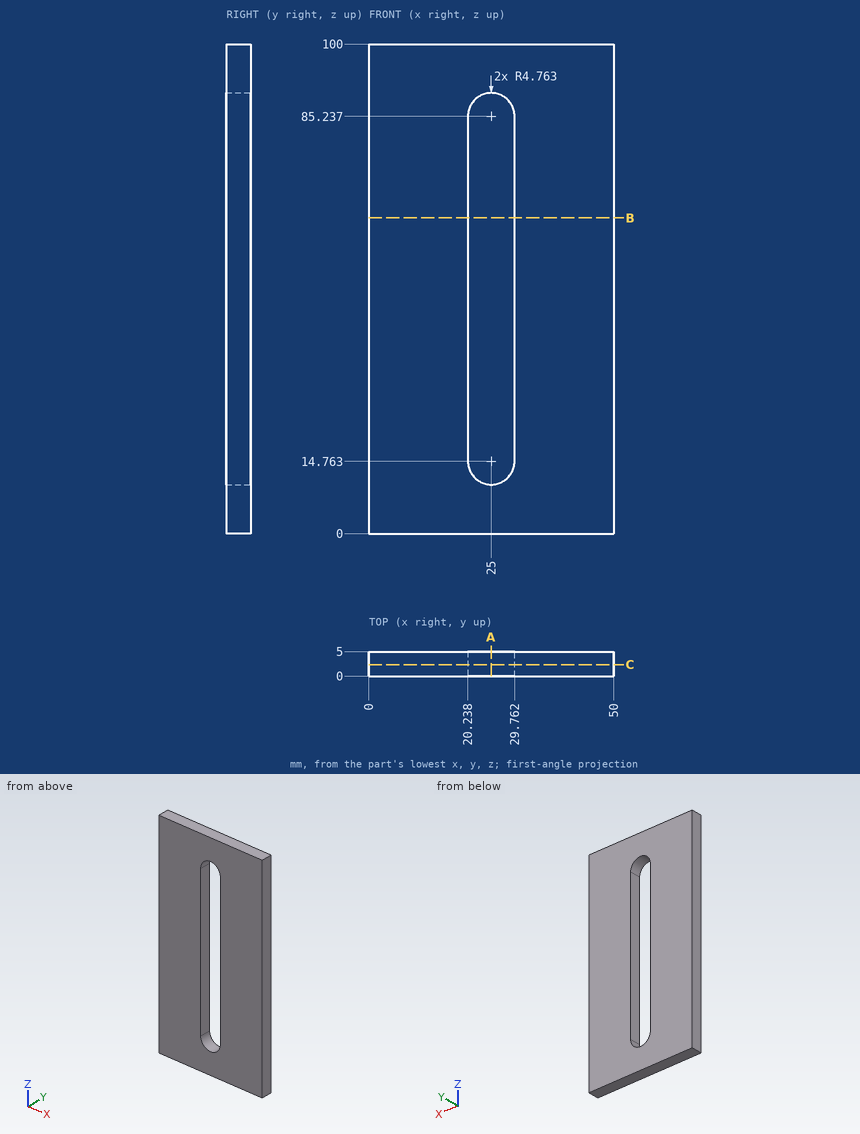
Geometry check sheet. Reference: drawing and pictorial views, mm from the part's lowest x, y, z. Round coordinates to 2 decimals unless told otherwise and drop trailing zeros. Order: outer loops, then holes, each group sorted by start corner. A loop starts at its lowest first (then second) coordinate and runs counter-clockwise, first axis right, second up. Notation, with made-up numbers: M -26,57 L 2,57 A15 cw 2,61 Z; hole C -22.5,9.5 d7. An arc over 180 degrees is marked long. Write item = value, one per line.
Q1. Section check C-C (y = 2.3). Enter the section's corners in (x, z) (1 decimal), plus the area to 3 significant figures.
Answer block:
outline = M 0,0 L 50,0 L 50,100 L 0,100 Z; hole M 20.2,14.8 A4.8 ccw 29.8,14.8 L 29.8,85.2 A4.8 ccw 20.2,85.2 Z
area = 4,260 mm^2
Q2. Scan lines: line 1 (X direction, y = 1.1, z = 48.5); line 2 (Z direction, x = 27, y = 3.4); line 3 (Z direction, x = 21, y = 3.7) (1 decimal). Record each from-to range of solid material in increasing order.
Answer block:
line_1 = 0 to 20.24, 29.76 to 50
line_2 = 0 to 10.44, 89.56 to 100
line_3 = 0 to 12.2, 87.8 to 100
Q3. Section check B-B (z = 64.5). Enter the section's corners in (x, y), plus the area to 3 significant figures.
Answer block:
outline = M 0,0 L 20.24,0 L 20.24,5 L 0,5 Z; M 29.76,0 L 50,0 L 50,5 L 29.76,5 Z
area = 202 mm^2
Q4. Section check A-A (x = 25). Enter the section's corners in (y, z), plus the area to 3 significant figures.
Answer block:
outline = M 0,0 L 5,0 L 5,10 L 0,10 Z; M 0,90 L 5,90 L 5,100 L 0,100 Z
area = 100 mm^2
